Can you work these out from the model? Positions are in its coordinate system, mm. A direction names the side the tool comes from. Give positions to 0.01 mm unless a question says otherwise; leave off trailing zeros. Loops run counter-clockwise (first coordinate to the right, second up) from the corner with the lowest first, then second, coordinate; pieces in that order, holes last. Notation, with made-up numbers: (-36, -10) - (-4, -10) arc R13 ccw to (-4, 8) - close; hole circle Ø10 at (84.5, -20). An arc over 180 degrees is marked (long way). Write item = value, one per line.
from build123d import *

# Parameters (mm, degrees)
SKETCH1_R           = 2.032
SKETCH1_R_2         = 4.7625
BOSS_EXTRUDE1_DEPTH = 3.175
FILLET1_R           = 6.35
SKETCH2_R           = 2.032
CUT_EXTRUDE1_DEPTH  = 116.854784776
FILLET2_R           = 2.3876
CUT_EXTRUDE2_REACH  = 117.855
FILLET3_R           = 3.175


with BuildPart() as part:
    # Sketch1 → Boss-Extrude1 (new body)
    with BuildSketch(Plane.XY):
        with BuildLine():
            Line((0, 0), (-99.21875, 0))
            Line((-99.21875, 0), (-99.21875, 25.4))
            ThreePointArc((-99.21875, 25.4), (-99.216112514, 25.559225204), (-99.208202949, 25.718275702))
            Line((-99.208202949, 25.718275702), (-97.583411312, 50.206818816))
            ThreePointArc((-97.583411312, 50.206818816), (-92.015151864, 58.871103506), (-81.820717516, 57.405207601))
            Line((-81.820717516, 57.405207601), (-64.992407125, 42.82279889))
            ThreePointArc((-64.992407125, 42.82279889), (-64.174703888, 41.906719209), (-63.615743119, 40.813374148))
            Line((-63.615743119, 40.813374148), (-58.084627995, 25.4))
            Line((-58.084627995, 25.4), (-3.297296565, 25.4))
            ThreePointArc((-3.297296565, 25.4), (0.195780415, 12.939434189), (0, 0))
        make_face()
        with Locations((-44.45, 7.14375)):
            Circle(SKETCH1_R, mode=Mode.SUBTRACT)
        with Locations((-84.089661312, 16.5735)):
            Circle(SKETCH1_R_2, mode=Mode.SUBTRACT)
        with Locations((-88.058411312, 50.206818816)):
            Circle(SKETCH1_R_2, mode=Mode.SUBTRACT)
        with Locations((-4.19910616, 6.35)):
            Circle(SKETCH1_R, mode=Mode.SUBTRACT)
        with Locations((-5.795027999, 19.05)):
            Circle(SKETCH1_R, mode=Mode.SUBTRACT)
        with Locations((-94.45625, 6.35)):
            Circle(SKETCH1_R, mode=Mode.SUBTRACT)
        with Locations((-94.45625, 19.05)):
            Circle(SKETCH1_R, mode=Mode.SUBTRACT)
    extrude(amount=BOSS_EXTRUDE1_DEPTH)

    # Fillet1
    fillet1_edges = [part.edges().sort_by_distance(p)[0] for p in [
        (-58.084627995, 25.4, 1.5875),
    ]]
    fillet(fillet1_edges, radius=FILLET1_R)

    # Sketch2 → Cut-Extrude1 (cut, through all)
    with BuildSketch(Plane.XY.offset(3.175)):
        with Locations((-68.140747312, 39.189568816)):
            Circle(SKETCH2_R)
    extrude(amount=-CUT_EXTRUDE1_DEPTH, mode=Mode.SUBTRACT)

    # Fillet2
    fillet2_edges = [part.edges().sort_by_distance(p)[0] for p in [
        (-99.21875, 0, 1.5875),
    ]]
    fillet(fillet2_edges, radius=FILLET2_R)

    # Sketch4 → Cut-Extrude2 (cut, up to next)
    with BuildSketch(Plane(origin=(0, 0, 0), x_dir=(-1, 0, 0), z_dir=(0, 0, -1)), mode=Mode.PRIVATE) as cut_extrude2_sk1:
        with BuildLine():
            Line((14.906243411, 20.25001426), (40.306243411, 20.25001426))
            ThreePointArc((40.306243411, 20.25001426), (38.03973616, 12.863437985), (37.591162137, 5.14998574))
            Line((37.591162137, 5.14998574), (12.191162137, 5.14998574))
            ThreePointArc((12.191162137, 5.14998574), (12.63973616, 12.863437985), (14.906243411, 20.25001426))
        make_face()
    cut_extrude2_tool1 = extrude(cut_extrude2_sk1.sketch, amount=-CUT_EXTRUDE2_REACH, mode=Mode.PRIVATE) & part.part
    # Sketch4 → Cut-Extrude2 (cut, up to next)
    with BuildSketch(Plane(origin=(0, 0, 0), x_dir=(-1, 0, 0), z_dir=(0, 0, -1)), mode=Mode.PRIVATE) as cut_extrude2_sk2:
        with BuildLine():
            Line((71.210862075, 28.952720027), (92.501475834, 25.698758848))
            ThreePointArc((92.501475834, 25.698758848), (93.814902604, 26.098604816), (94.325334391, 27.37313456))
            Line((94.325334391, 27.37313456), (93.375138804, 41.6942974))
            ThreePointArc((93.375138804, 41.6942974), (92.556554604, 42.979979171), (91.032400998, 42.983652428))
            Line((91.032400998, 42.983652428), (70.691982826, 31.916450766))
            ThreePointArc((70.691982826, 31.916450766), (69.886987798, 30.248228031), (71.210862075, 28.952720027))
        make_face()
    cut_extrude2_tool2 = extrude(cut_extrude2_sk2.sketch, amount=-CUT_EXTRUDE2_REACH, mode=Mode.PRIVATE) & part.part
    # Sketch4 → Cut-Extrude2 (cut, up to next)
    with BuildSketch(Plane(origin=(0, 0, 0), x_dir=(-1, 0, 0), z_dir=(0, 0, -1)), mode=Mode.PRIVATE) as cut_extrude2_sk3:
        with BuildLine():
            Line((73.81875, 5.14998574), (51.59375, 5.14998574))
            ThreePointArc((51.59375, 5.14998574), (51.145175977, 12.863437985), (48.878668725, 20.25001426))
            Line((48.878668725, 20.25001426), (70.807625266, 20.25001426))
            ThreePointArc((70.807625266, 20.25001426), (73.317974303, 12.900366376), (73.81875, 5.14998574))
        make_face()
    cut_extrude2_tool3 = extrude(cut_extrude2_sk3.sketch, amount=-CUT_EXTRUDE2_REACH, mode=Mode.PRIVATE) & part.part
    add(cut_extrude2_tool1.solids().sort_by_distance((-25.621324, 12.7, 0))[0], mode=Mode.SUBTRACT)
    add(cut_extrude2_tool2.solids().sort_by_distance((-84.934877, 33.097306, 0))[0], mode=Mode.SUBTRACT)
    add(cut_extrude2_tool3.solids().sort_by_distance((-61.941303, 12.68386, 0))[0], mode=Mode.SUBTRACT)

    # Fillet3
    fillet3_edges = [part.edges().sort_by_distance(p)[0] for p in [
        (-70.807625266, 20.25001426, 1.5875),
        (-73.81875, 5.14998574, 1.5875),
        (-51.59375, 5.14998574, 1.5875),
        (-48.878668725, 20.25001426, 1.5875),
        (-40.306243411, 20.25001426, 1.5875),
        (-37.591162137, 5.14998574, 1.5875),
        (-12.191162137, 5.14998574, 1.5875),
        (-14.906243411, 20.25001426, 1.5875),
    ]]
    fillet(fillet3_edges, radius=FILLET3_R)


solid = part.part
Q1. Imagine slicing it at D-D, the plane z = 0.9. Give the number of separate pieces and of enclosed holes in the cut face, then the cut area to 3 significant figures.
Output:
separate_pieces = 1
enclosed_holes = 11
area = 2,360 mm2
Q2. For pin 1 (1 mm diameter, centred on x = -22, z = 1, fed in from +Y); pin 2 (3.5 mm diameter, centred on x = -5.8, y = 19.05, fed in from +Z), each with a flat end and sliding along its axis, tell me the tip position at first contact or that it passes through.
Output:
pin_1 = 25.4
pin_2 = through
Q3. Imagine slicing it at C-C, the plane x = -84.5. Write out the boundary of the cut face in (y, z) (3 decimals).
Output:
outline = (0, 0) - (11.829, 0) - (11.829, 3.175) - (0, 3.175) - close; (21.318, 0) - (26.922, 0) - (26.922, 3.175) - (21.318, 3.175) - close; (39.429, 0) - (47.042, 0) - (47.042, 3.175) - (39.429, 3.175) - close; (53.372, 0) - (59.042, 0) - (59.042, 3.175) - (53.372, 3.175) - close
Q4. I need wall thicknesses on L1, parallel to Y at x = -84, z = 0.6; L2, parallel to Y at x = -19, z = 3.05; L3, parallel to X at y = 7, z = 0.1. Which ranges of each line are inside material? Lowest first, please.
Output:
L1 = 0 to 11.81, 21.34 to 27, 39.16 to 47.71, 52.7 to 58.82
L2 = 0 to 5.15, 20.25 to 25.4
L3 = -99.22 to -96.38, -92.53 to -73.57, -51.93 to -46.48, -42.42 to -37.26, -12.44 to -6.12, -2.27 to 0.57
Q5. Imagine slicing it at A-A, the plane x = -44.45. Write out the boundary of the cut face in (y, z) (3 decimals).
Output:
outline = (0, 0) - (5.112, 0) - (5.112, 3.175) - (0, 3.175) - close; (9.176, 0) - (25.4, 0) - (25.4, 3.175) - (9.176, 3.175) - close
Q6. Imagine slicing it at B-B, the plane y = 53.5. Write out the boundary of the cut face in (x, z) (3 decimals), then the cut area to 3 significant figures.
Output:
outline = (-96.996, 0) - (-91.499, 0) - (-91.499, 3.175) - (-96.996, 3.175) - close; (-84.618, 0) - (-77.314, 0) - (-77.314, 3.175) - (-84.618, 3.175) - close
area = 40.6 mm2
Q7. We'd pull the mould along X, two halves only. Please class faces 3 (the flat face through (-48, 0, 2)), 4 (the cylindrical face through (-57.23, 26.53, 1.61)), 5 (the flat face through (-99.219, 14, 2)), 6 (the flat face through (-81.71, 27.35, 1.57)): released by +X, released by -X, zero draft, split by the parting line, or undercut.
Output:
face_3 = zero draft
face_4 = released by +X
face_5 = released by -X
face_6 = undercut
Q8. Which directions (+Z, -Z, +X, -X, +Y, -Y) give clear straight access to the entire face, cutting with the end or side of a thin tool? Please do faces 1 (the flat face through (-60, 24, 3.175)), 2 (the cylindrical face through (-73.185, 13.533, 1.565)).
Output:
face_1 = +Z, +X, -X, +Y, -Y
face_2 = +Z, -Z
